Build history of the part. All positions in model axes, mm. Give positions to 0.01 mm unless a question says otherwise; leave off trailing zeros. Loops run counter-clockwise (first coordinate to the right, second up) from the corner with the lowest first, then second, coordinate; pieces in that order, holes last. Notation, with made-up numbers: (47, 6) -> (59, 6) arc R23 ccw to (59, 39) -> close; hole circle Ø7 at (41, 63.25). An arc over 180 degrees is marked (long way). Answer in a Markdown table with one row per item. Add a question column.
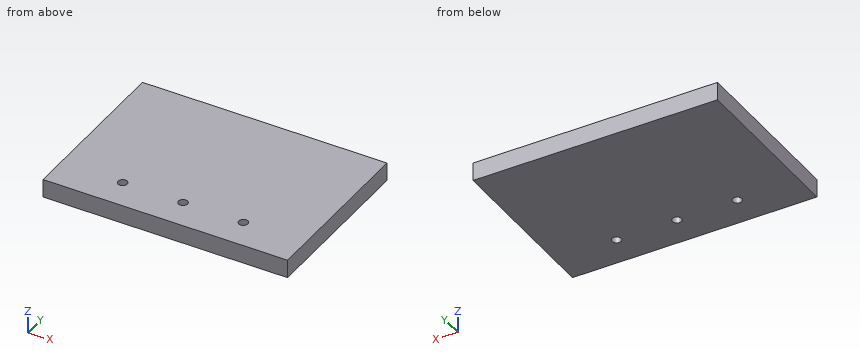
Autodesk Inventor part; units mm, degrees
ref_plane "YZ Plane" through (0, 0, 0) normal (1, 0, 0) x (0, 1, 0)
ref_plane "XZ Plane" through (0, 0, 0) normal (0, 1, 0) x (-1, 0, 0)
ref_plane "XY Plane" through (0, 0, 0) normal (0, 0, 1) x (1, 0, 0)
sketch "Sketch1" plane through (0, 0, 0) normal (0, 0, 1) x (1, 0, 0)
  line L0 (0, 0) -> (0, 40)
  line L1 (0, 40) -> (0, 46)
  line L2 (0, 46) -> (40, 46)
  line L3 (40, -10) -> (0, -10)
  line L4 (0, -10) -> (0, 0)
  line L5 (40, 46) -> (40, 40)
  line L6 (40, 40) -> (40, -10)
  line L7 (0, 40) -> (40, 40) construction
  line L8 (0, 0) -> (19.75, 0) construction
  dimension "d0" = 40
  dimension "d1" = 6
  dimension "d2" = 10
  dimension "d3" = 40
  dimension "d4" = 40
  dimension "d5" = 19.75
extrude "Extrusion1" add sketch "Sketch1" along normal blind 6
fillet "Fillet1" [suppressed]
hole "Hole1" at (0, 0, 0) at (19.75, 0, 0) direction (0, 0, 1) diameter 3 end through all
mirror "Mirror1" about plane through (0, 40, 0) normal (-1, 0, 0)
properties part number "segment0a" material "Plywood, Finish"
(1) Flat gauge pin, fed straight in: pin 1 Ø1.8 at (x, y) = (19.75, 0) entering from -Z. Where does the tip first touch, or does it go through?
(2) Saw through at A-A, the plane y = 0. List the corners of the cut face in (x, z), then the cut area to 3 significant figures.
(3) Saw through at B-B, the plane x = 19.75. List the corners of the cut face in (y, z).
(4) Wall check: line 1 along X through (y, z) = (0, 2.6); line 2 along Y through (x, z) = (0, 2.55); line 3 along Y through (x, z) = (21, 2.4). Give the ranges that are in metal, low to high. Write a range as from..to.
Worked answers:
| question | item | result |
|---|---|---|
| 1 | pin 1 | through |
| 2 | outline | (-40, 0) -> (-21.25, 0) -> (-21.25, 6) -> (-40, 6) -> close; (-18.25, 0) -> (-1.5, 0) -> (-1.5, 6) -> (-18.25, 6) -> close; (1.5, 0) -> (18.25, 0) -> (18.25, 6) -> (1.5, 6) -> close; (21.25, 0) -> (40, 0) -> (40, 6) -> (21.25, 6) -> close |
| 2 | area | 426 mm^2 |
| 3 | outline | (-10, 0) -> (-1.5, 0) -> (-1.5, 6) -> (-10, 6) -> close; (1.5, 0) -> (46, 0) -> (46, 6) -> (1.5, 6) -> close |
| 4 | line 1 | -40..-21.25, -18.25..-1.5, 1.5..18.25, 21.25..40 |
| 4 | line 2 | -10..-1.5, 1.5..46 |
| 4 | line 3 | -10..-0.83, 0.83..46 |
